Geometry: final body of the model. Coordinates: model frame, mm. A direction names the side the tool comes from. Give positions to 0.01 mm unless a question says otherwise; leave off trailing zeros. Write each loop counter-clockwise with the first axis right and the second up, starting at its lowest first coordinate (ties: lowest second). Pieces come first, ordered by that corner, then holes. Notation, with made-up numbers: (7, 71.25) - (29, 71.25) arc R17 ccw to (29, 77.25) - close; hole circle Ø4 at (52.25, 26.5). An arc over 180 degrees is marked (long way). Return JSON: item names as keys, results as strings.
from build123d import *

# Parameters (mm, degrees)
SKETCH_W    = 200
SKETCH_H    = 90
SKETCH_R    = 1.5625
PAD_DEPTH   = 12
FILLET_R    = 30
FILLET001_R = 3


with BuildPart() as part:
    # Sketch → Pad (new body)
    with BuildSketch(Plane.XY):
        with Locations((100, -45)):
            Rectangle(SKETCH_W, SKETCH_H)
        with Locations((175, -10)):
            Circle(SKETCH_R, mode=Mode.SUBTRACT)
        with Locations((175, -30)):
            Circle(SKETCH_R, mode=Mode.SUBTRACT)
        with Locations((185, -20)):
            Circle(SKETCH_R, mode=Mode.SUBTRACT)
        with Locations((185, -40)):
            Circle(SKETCH_R, mode=Mode.SUBTRACT)
        with Locations((25, -10)):
            Circle(SKETCH_R, mode=Mode.SUBTRACT)
        with Locations((25, -30)):
            Circle(SKETCH_R, mode=Mode.SUBTRACT)
        with Locations((15, -20)):
            Circle(SKETCH_R, mode=Mode.SUBTRACT)
        with Locations((15, -40)):
            Circle(SKETCH_R, mode=Mode.SUBTRACT)
        with Locations((185, -10)):
            Circle(SKETCH_R, mode=Mode.SUBTRACT)
        with Locations((175, -20)):
            Circle(SKETCH_R, mode=Mode.SUBTRACT)
        with Locations((185, -30)):
            Circle(SKETCH_R, mode=Mode.SUBTRACT)
        with Locations((175, -40)):
            Circle(SKETCH_R, mode=Mode.SUBTRACT)
        with Locations((15, -10)):
            Circle(SKETCH_R, mode=Mode.SUBTRACT)
        with Locations((25, -20)):
            Circle(SKETCH_R, mode=Mode.SUBTRACT)
        with Locations((15, -30)):
            Circle(SKETCH_R, mode=Mode.SUBTRACT)
        with Locations((25, -40)):
            Circle(SKETCH_R, mode=Mode.SUBTRACT)
        with BuildLine():
            ThreePointArc((158.0113, -7.9887), (155.0113, -4.9887), (152.0113, -7.9887))
            Line((152.0113, -7.9887), (152.0113, -17.9887))
            ThreePointArc((152.0113, -17.9887), (155.0113, -20.9887), (158.0113, -17.9887))
            Line((158.0113, -7.9887), (158.0113, -17.9887))
        make_face(mode=Mode.SUBTRACT)
        with BuildLine():
            ThreePointArc((151, -31.5), (131.5, -12), (112, -31.5))
            Line((112, -31.5), (112, -41.5))
            ThreePointArc((112, -41.5), (131.5, -61), (151, -41.5))
            Line((151, -31.5), (151, -41.5))
        make_face(mode=Mode.SUBTRACT)
        with BuildLine():
            ThreePointArc((158.0113, -55.0113), (155.0113, -52.0113), (152.0113, -55.0113))
            Line((152.0113, -55.0113), (152.0113, -65.0113))
            ThreePointArc((152.0113, -65.0113), (155.0113, -68.0113), (158.0113, -65.0113))
            Line((158.0113, -55.0113), (158.0113, -65.0113))
        make_face(mode=Mode.SUBTRACT)
        with BuildLine():
            ThreePointArc((110.9887, -55.0113), (107.9887, -52.0113), (104.9887, -55.0113))
            Line((104.9887, -55.0113), (104.9887, -65.0113))
            ThreePointArc((104.9887, -65.0113), (107.9887, -68.0113), (110.9887, -65.0113))
            Line((110.9887, -55.0113), (110.9887, -65.0113))
        make_face(mode=Mode.SUBTRACT)
        with BuildLine():
            ThreePointArc((110.9887, -7.9887), (107.9887, -4.9887), (104.9887, -7.9887))
            Line((104.9887, -7.9887), (104.9887, -17.9887))
            ThreePointArc((104.9887, -17.9887), (107.9887, -20.9887), (110.9887, -17.9887))
            Line((110.9887, -7.9887), (110.9887, -17.9887))
        make_face(mode=Mode.SUBTRACT)
    extrude(amount=PAD_DEPTH)

    # Fillet
    fillet_edges = [part.edges().sort_by_distance(p)[0] for p in [
        (0, -90, 6),
        (200, -90, 6),
    ]]
    fillet(fillet_edges, radius=FILLET_R)

    # Fillet001
    fillet001_edges = [part.edges().sort_by_distance(p)[0] for p in [
        (200, 0, 6),
        (0, 0, 6),
    ]]
    fillet(fillet001_edges, radius=FILLET001_R)


solid = part.part
Q1. Material intervals for probe 1 along Y at (x, z) = (25, 3); probe 2 along X at (y, z) = (-8, 10.5); probe 3 along X at (y, z) = (-17, 7.75), sorted ascending. Write a range as [from, to].
Answer key:
{"probe 1": "y = [-89.58, -41.56], [-38.44, -31.56], [-28.44, -21.56], [-18.44, -11.56], [-8.44, 0]", "probe 2": "x = [0, 104.99], [110.99, 152.01], [158.01, 200]", "probe 3": "x = [0, 104.99], [110.99, 118.46], [144.54, 152.01], [158.01, 200]"}
Q2. Mould query, pull axis X, two halves, no side actions, for faces 1 (the flat face through (99, -90, 6)), 2 (the flat face through (0, -32, 6)), 3 (the flat face through (110.989, -60, 6)). Classes: pulls with the +X half, pulls with the -X half, needs draft (parallel to the pull), parting line crosses it, or undercut.
Answer key:
{"face 1": "needs draft", "face 2": "pulls with the -X half", "face 3": "undercut"}
Q3. Section query B-B, the plane x = 131.5. Return the cut outline in (y, z), plus the area to 3 significant figures.
Answer key:
{"outline": "(-90, 0) - (-61, 0) - (-61, 12) - (-90, 12) - close; (-12, 0) - (0, 0) - (0, 12) - (-12, 12) - close", "area": "492 mm^2"}
Q4. Set-up query: faces 4 (the cylindrical face through (131.071, -60.995, 5.916)), 5 (the flat face through (99, -44, 0)). Return all of +Z, -Z, +X, -X, +Y, -Y with unobstructed straight access to the full face (end or side cutting, diameter ignored); none if empty.
Answer key:
{"face 4": "+Z, -Z", "face 5": "-Z, +X, -X, +Y, -Y"}
Q5. Section query D-D, the plane x = 20.5. Return the cut outline in (y, z), plus the area to 3 significant figures.
Answer key:
{"outline": "(-88.46, 0) - (0, 0) - (0, 12) - (-88.46, 12) - close", "area": "1,060 mm^2"}
Q6. Pin query (flat end, axial travel): P1, Ø2.5, axis at x = 185, y = -40, coming from the -Z side; P2, Ø5, axis at y = -76, z = 5.5, coming from the -X side; P3, Ø6, axis at y = -64.5, z = 9, coming from the -X side. Return the tip coordinate at first contact, or that it passes through.
Answer key:
{"P1": "passes through", "P2": "stops at x = 3.21", "P3": "stops at x = 0.04"}
Q7. Section query A-A, the plane y = -36. Return the cut outline in (x, z), plus the area to 3 significant figures.
Answer key:
{"outline": "(0, 0) - (112, 0) - (112, 12) - (0, 12) - close; (151, 0) - (200, 0) - (200, 12) - (151, 12) - close", "area": "1,930 mm^2"}
Q8. Section query C-C, the plane z = 6.5. Count the separate pieces of the cut face and the enclosed holes in it, plus the area to 3 significant figures.
Answer key:
{"separate pieces": "1", "enclosed holes": "21", "area": "15,500 mm^2"}
